Read the model definition and answer for the solid it produces. Units are mm, in the model's axes. A direction names the side the tool comes from. Coordinates: 2 decimals unless noted, no trailing zeros. Write each loop counter-clockwise with the first axis right and the second up, starting at its lowest first coordinate (ties: lowest second). Pieces come first, ordered by that corner, then holes.
1) Each of these flat-tipped pins is pushed along its axis until it touches: pin 1 Ø5.5 at (x, z) = (2.413, -5.08) entering from +Y; pin 2 Ø1 at (x, y) = (12, 31.5) entering from +Z (3 decimals); pin 3 Ø0.9 at (x, z) = (-1.5, -7.5) entering from -Y. Where does it stop, or does it pass through?
2) The part is cut by section D-D (z = -8.75). Determine the outline of the cut face in (x, y), then the cut area to 3 significant figures.
3) The part is cut by section A-A (z = -5.08). Determine the outline of the cut face in (x, y) (3 decimals), then the cut area to 3 significant figures.
4) The part is cut by section B-B (y = 9). Determine the outline of the cut face in (x, z).
5) The part is cut by section C-C (x = 16). Determine the outline of the cut face in (y, z).
6) Determine the mould class of faces 5 (the face through (12, 31, -4.572)), 6 (the face through (10.795, 31, -5)), 7 (the face through (2.92, 0, -3.88)), 8 (the face through (10.475, 29.071, -3.208)) for opening direction Z: +Z half, -Z half, draft (parallel to the pull), parting line (faces both ways), or undercut.
7) Find the intervals of material crossed by line 1 (X direction, y = 31.1, z = -5.08) (3 decimals); line 2 (Y direction, x = 14, z = -7.75); line 3 (X direction, y = 15.5, z = -5), in increasing order.
8) Which of the six approach directions +Z, -Z, +X, -X, +Y, -Y give full straight-line access (tool end or side, diameter ignored) to faces 1 (the face through (-2, 27.432, -5)), 2 (the face through (4.826, 30, -5)), 3 (the face through (4.075, 3.133, -6.477)), 4 (the face through (1, 30.734, -4))?
from build123d import *

# Parameters (mm, degrees)
SKETCH1_W           = 14.732
SKETCH1_H           = 10.922
BOSS_EXTRUDE1_DEPTH = 10.16
SKETCH2_R           = 1.143
CUT_EXTRUDE1_DEPTH  = 40.068139551
CUT_EXTRUDE2_DEPTH  = 1.524
CUT_EXTRUDE5_START  = -1.524
SKETCH5_R           = 1.143
CUT_EXTRUDE5_DEPTH  = 1.524
SKETCH6_R           = 2.54
BOSS_EXTRUDE2_DEPTH = 1.778
SKETCH7_R           = 1.905
BOSS_EXTRUDE3_DEPTH = 2.032
SKETCH9_W           = 2.794
SKETCH9_H           = 1.016
CUT_EXTRUDE6_DEPTH  = 2.032


with BuildPart() as part:
    # Sketch1 → Boss-Extrude1 (new body)
    with BuildSketch(Plane.XY):
        with Locations((12.192, 22.733)):
            Rectangle(SKETCH1_W, SKETCH1_H)
        Polygon((-3.048, 27.432), (0, 27.432), (0, 0), (4.826, 0), (4.826, 32.258), (-3.048, 32.258), align=None)
    extrude(amount=-BOSS_EXTRUDE1_DEPTH)

    # Sketch2 → Cut-Extrude1 (cut, through all)
    with BuildSketch(Plane(origin=(0, 0, 0), x_dir=(-1, 0, 0), z_dir=(0, -1, 0))):
        with Locations(Location((-2.413, 5.08, 0), (0, 0, 90))):
            Circle(SKETCH2_R)
    extrude(amount=-CUT_EXTRUDE1_DEPTH, mode=Mode.SUBTRACT)

    # Sketch3 → Cut-Extrude2 (cut)
    with BuildSketch(Plane(origin=(4.826, 0, 0), x_dir=(0, 0, -1), z_dir=(1, 0, 0))):
        with BuildLine():
            Line((10.16, 1.27), (8.382, 1.27))
            ThreePointArc((8.382, 1.27), (6.477, 3.175), (8.382, 5.08))
            Line((8.382, 5.08), (10.16, 5.08))
            Line((10.16, 5.08), (10.16, 1.27))
        make_face()
    extrude(amount=-CUT_EXTRUDE2_DEPTH, mode=Mode.SUBTRACT)

    # Sketch5 → Cut-Extrude5 (cut)
    with BuildSketch(Plane(origin=(0, 32.258, 0), x_dir=(1, 0, 0), z_dir=(0, 1, 0)).offset(CUT_EXTRUDE5_START)):
        with BuildLine():
            Line((4.826, 3.175), (4.826, 5.08))
            Line((4.826, 5.08), (4.826, 6.985))
            ThreePointArc((4.826, 6.985), (-0.661344483, 5.08), (4.826, 3.175))
        make_face()
        with Locations(Location((2.413, 5.08, 0), (0, 0, 90))):
            Circle(SKETCH5_R, mode=Mode.SUBTRACT)
    extrude(amount=CUT_EXTRUDE5_DEPTH, mode=Mode.SUBTRACT)

    # Sketch6 → Boss-Extrude2 (add)
    with BuildSketch(Plane(origin=(0, 28.194, 0), x_dir=(1, 0, 0), z_dir=(0, 1, 0))):
        with Locations(Location((12.192, 5.08, 0), (0, 0, 90))):
            Circle(SKETCH6_R)
    extrude(amount=BOSS_EXTRUDE2_DEPTH)

    # Sketch7 → Boss-Extrude3 (add)
    with BuildSketch(Plane(origin=(0, 29.972, 0), x_dir=(1, 0, 0), z_dir=(0, 1, 0))):
        with Locations(Location((12.192, 5.08, 0), (0, 0, 270))):
            Circle(SKETCH7_R)
    extrude(amount=BOSS_EXTRUDE3_DEPTH)

    # Sketch9 → Cut-Extrude6 (cut)
    with BuildSketch(Plane(origin=(0, 32.004, 0), x_dir=(1, 0, 0), z_dir=(0, 1, 0))):
        with Locations((12.192, 5.08)):
            Rectangle(SKETCH9_W, SKETCH9_H)
    extrude(amount=-CUT_EXTRUDE6_DEPTH, mode=Mode.SUBTRACT)


solid = part.part
Reported:
1. pin 1: stops at y = 30.73
1. pin 2: stops at z = -3.175
1. pin 3: stops at y = 27.43
2. outline: (-3.05, 27.43) - (0, 27.43) - (0, 0) - (4.83, 0) - (4.83, 1.27) - (3.3, 1.27) - (3.3, 5.08) - (4.83, 5.08) - (4.83, 17.27) - (19.56, 17.27) - (19.56, 28.19) - (4.83, 28.19) - (4.83, 32.26) - (-3.05, 32.26) - close
2. area: 325 mm2
3. outline: (-3.048, 27.432) - (0, 27.432) - (0, 0) - (1.27, 0) - (1.27, 30.734) - (-0.661, 30.734) - (-0.661, 32.258) - (-3.048, 32.258) - close; (3.556, 0) - (4.826, 0) - (4.826, 17.272) - (19.558, 17.272) - (19.558, 28.194) - (14.732, 28.194) - (14.732, 29.972) - (14.097, 29.972) - (14.097, 32.004) - (13.589, 32.004) - (13.589, 29.972) - (10.795, 29.972) - (10.795, 32.004) - (10.287, 32.004) - (10.287, 29.972) - (9.652, 29.972) - (9.652, 28.194) - (4.826, 28.194) - (4.826, 30.734) - (3.556, 30.734) - close
3. area: 264 mm2
4. outline: (0, -10.16) - (4.83, -10.16) - (4.83, 0) - (0, 0) - close; hole circle Ø2.29 at (2.41, -5.08)
5. outline: (17.27, -10.16) - (28.19, -10.16) - (28.19, 0) - (17.27, 0) - close
6. face 5: undercut
6. face 6: undercut
6. face 7: draft
6. face 8: parting line
7. line 1: x = -3.048 to -0.661, 10.287 to 10.795, 13.589 to 14.097
7. line 2: y = 17.27 to 28.19
7. line 3: x = 0 to 1.27, 3.55 to 4.83
8. face 1: +Z, -Z, -X, -Y
8. face 2: +Z, -Z, +Y
8. face 3: -Z, +X
8. face 4: +Y
